The listing builds one solid part. Answer for the finished solid, in the listing's coordinates (mm). Round coordinates to 2 decimals unless told otherwise and drop trailing zeros. Write each loop counter-clockwise with the first axis right and the second up, starting at its lowest first coordinate (ties: lowest second). Pieces come first, ordered by that corner, then holes. Notation, with made-up numbers: (-24, 45.25) - (7, 45.25) arc R22 cw to (7, 81.25) - close; hole circle Ø4 at (66, -40). An arc over 180 degrees is marked (long way). Return JSON: item names as keys, results as strings. Group by question number.
(1) Section A-A, the plane x = -20.5 is taken. Write down the section's boundary in (y, z), then the cut area to 3 significant figures.
(2) Section D-D, the plane x = -86.5 is taken. Write down the section's boundary in (y, z), then the cut area to 3 significant figures.
(3) Section B-B, the plane y = 6.5 is taken. Write down the section's boundary in (x, z), then the cut area to 3 significant figures.
(4) Section C-C, the plane z = 0.4 is taken. Give the number of separate pieces and of enclosed holes in the cut face, then the cut area to 3 significant figures.
(5) Find the intervals of material crossed by line 1 along Y through (x, z) = (44.5, 0.2); line 2 along Y through (x, z) = (-47, 1.4); line 3 along X through (y, z) = (-12, 0.35), in increasing order. Write a range as [from, to].
(6) Each of these flat-tipped pins is pushed along its axis until it touches: pin 1 (3.5 mm diameter, centred on x = -20.5, y = 6.5, fed in from +Z); pin 2 (8 mm diameter, centred on x = -86.5, y = 6.5, fed in from -Z); pin 3 (0.8 mm diameter, centred on x = 65.5, z = 0.5, fed in from -Y). Where does it stop, or does it pass through?
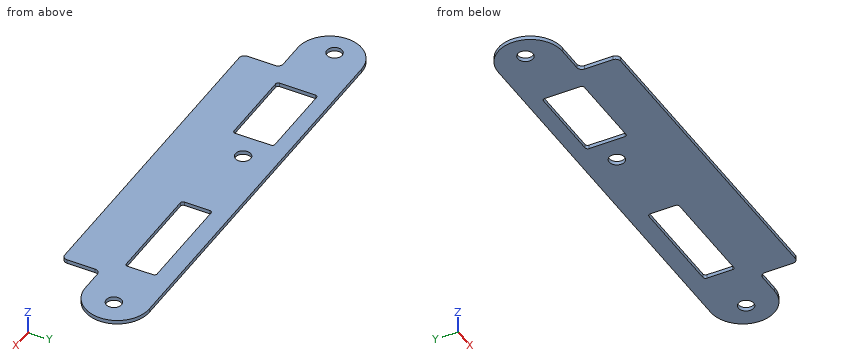
```python
from build123d import *

# Parameters (mm, degrees)
ESQUISSE1_R      = 3
EXTRUSION1_DEPTH = 1.5


with BuildPart() as part:
    # Esquisse1 → Extrusion1 (new body)
    with BuildSketch(Plane.XY):
        with BuildLine():
            Line((-83, -6), (-72.5, -6))
            ThreePointArc((-72.5, -6), (-71.085786438, -6.585786438), (-70.5, -8))
            Line((-70.5, -8), (-70.5, -19))
            ThreePointArc((-70.5, -19), (-69.914213562, -20.414213562), (-68.5, -21))
            Line((-68.5, -21), (57.5, -21))
            ThreePointArc((57.5, -21), (58.914213562, -20.414213562), (59.5, -19))
            Line((59.5, -19), (59.5, -8))
            ThreePointArc((59.5, -8), (60.085786438, -6.585786438), (61.5, -6))
            Line((61.5, -6), (70.25, -6))
            ThreePointArc((70.25, -6), (82.75, 6.5), (70.25, 19))
            Line((70.25, 19), (-83, 19))
            ThreePointArc((-83, 19), (-95.5, 6.5), (-83, -6))
        make_face()
        with Locations((-86.5, 6.5)):
            Circle(ESQUISSE1_R, mode=Mode.SUBTRACT)
        with Locations((-20.5, 6.5)):
            Circle(ESQUISSE1_R, mode=Mode.SUBTRACT)
        with Locations((72.75, 6.5)):
            Circle(ESQUISSE1_R, mode=Mode.SUBTRACT)
        with BuildLine():
            Line((-31.5, 13), (-61.5, 13))
            ThreePointArc((-61.5, 13), (-62.207106781, 12.707106781), (-62.5, 12))
            Line((-62.5, 12), (-62.5, -2))
            ThreePointArc((-62.5, -2), (-62.207106781, -2.707106781), (-61.5, -3))
            Line((-61.5, -3), (-31.5, -3))
            ThreePointArc((-31.5, -3), (-30.792893219, -2.707106781), (-30.5, -2))
            Line((-30.5, -2), (-30.5, 12))
            ThreePointArc((-30.5, 12), (-30.792893219, 12.707106781), (-31.5, 13))
        make_face(mode=Mode.SUBTRACT)
        with BuildLine():
            Line((51.75, 12), (12.75, 12))
            ThreePointArc((12.75, 12), (12.042893219, 11.707106781), (11.75, 11))
            Line((11.75, 11), (11.75, 1))
            ThreePointArc((11.75, 1), (12.042893219, 0.292893219), (12.75, 0))
            Line((12.75, 0), (51.75, 0))
            ThreePointArc((51.75, 0), (52.457106781, 0.292893219), (52.75, 1))
            Line((52.75, 1), (52.75, 11))
            ThreePointArc((52.75, 11), (52.457106781, 11.707106781), (51.75, 12))
        make_face(mode=Mode.SUBTRACT)
    extrude(amount=EXTRUSION1_DEPTH)


solid = part.part
```
Working result:
{
 "1": {"outline": "(-21, 0) - (3.5, 0) - (3.5, 1.5) - (-21, 1.5) - close; (9.5, 0) - (19, 0) - (19, 1.5) - (9.5, 1.5) - close", "area": "51.0 mm^2"},
 "2": {"outline": "(-5.5, 0) - (3.5, 0) - (3.5, 1.5) - (-5.5, 1.5) - close; (9.5, 0) - (18.5, 0) - (18.5, 1.5) - (9.5, 1.5) - close", "area": "27.0 mm^2"},
 "3": {"outline": "(-95.5, 0) - (-89.5, 0) - (-89.5, 1.5) - (-95.5, 1.5) - close; (-83.5, 0) - (-62.5, 0) - (-62.5, 1.5) - (-83.5, 1.5) - close; (-30.5, 0) - (-23.5, 0) - (-23.5, 1.5) - (-30.5, 1.5) - close; (-17.5, 0) - (11.75, 0) - (11.75, 1.5) - (-17.5, 1.5) - close; (52.75, 0) - (69.75, 0) - (69.75, 1.5) - (52.75, 1.5) - close; (75.75, 0) - (82.75, 0) - (82.75, 1.5) - (75.75, 1.5) - close", "area": "131 mm^2"},
 "4": {"separate pieces": "1", "enclosed holes": "5", "area": "5,190 mm^2"},
 "5": {"line 1": "y = [-21, 0], [12, 19]", "line 2": "y = [-21, -3], [13, 19]", "line 3": "x = [-70.5, 59.5]"},
 "6": {"pin 1": "passes through", "pin 2": "stops at z = 0", "pin 3": "stops at y = -6"}
}
